```python
from build123d import *

# Parameters (mm, degrees)
SKETCH_1_W                    = 68
SKETCH_1_H                    = 75
EXTRUDE_1_DEPTH               = 14
SKETCH_2_R                    = 8.25
CUT_EXTRUDE_1_DEPTH           = 53.519044165
SKETCH_6_R                    = 35
CUT_EXTRUDE_3_DEPTH           = 8
HOLE_WIZARD_M2_2_D            = 2.4
HOLE_WIZARD_M2_2_DEPTH        = 6.35
HOLE_WIZARD_M2_2_CSINK_D      = 4.4
HOLE_WIZARD_M2_2_CSINK_ANGLE  = 90
HOLE_WIZARD_M2_2_TIP          = 0.721032743
HOLE_WIZARD_M2_5_1_AT_2_COUNT = 2
HOLE_WIZARD_M2_5_1_AT_2_PITCH = 18.5
HOLE_WIZARD_M2_5_2_D          = 2.05
HOLE_WIZARD_M2_5_2_DEPTH      = 6.35
HOLE_WIZARD_M2_5_2_TIP        = 0.615882135
SKETCH_19_R                   = 5
CUT_EXTRUDE_5_DEPTH           = 52.246951129
HOLE_WIZARD_M3_1_D            = 3.4
HOLE_WIZARD_M3_1_CSINK_D      = 6.3
HOLE_WIZARD_M3_1_CSINK_ANGLE  = 90


with BuildPart() as part:
    # 草圖1 → 填料-伸長1 (new body)
    with BuildSketch(Plane.XY):
        Rectangle(SKETCH_1_W, SKETCH_1_H)
    extrude(amount=EXTRUDE_1_DEPTH)

    # 草圖2 → 除料-伸長1 (cut, through all)
    with BuildSketch(Plane(origin=(0, 0, 0), x_dir=(-1, 0, 0), z_dir=(0, 0, -1))):
        with Locations((0, -5)):
            Circle(SKETCH_2_R)
    extrude(amount=-CUT_EXTRUDE_1_DEPTH, mode=Mode.SUBTRACT)

    # 草圖6 → 除料-伸長3 (cut)
    with BuildSketch(Plane(origin=(0, 0, 0), x_dir=(-1, 0, 0), z_dir=(0, 0, -1))):
        with Locations((0, -5)):
            Circle(SKETCH_6_R)
    extrude(amount=-CUT_EXTRUDE_3_DEPTH, mode=Mode.SUBTRACT)

    # M2 錐坑平頭螺釘的錐孔2
    with Locations(Plane(origin=(0, 0, 8), x_dir=(-1, 0, 0), z_dir=(0, 0, -1))):
        with Locations((-7.5, 2.5), (7.5, -12.5), (-7.5, -12.5), (7.5, 2.5)):
            CounterSinkHole(HOLE_WIZARD_M2_2_D / 2, HOLE_WIZARD_M2_2_CSINK_D / 2, depth=HOLE_WIZARD_M2_2_DEPTH, counter_sink_angle=HOLE_WIZARD_M2_2_CSINK_ANGLE)
            with Locations((0, 0, -(HOLE_WIZARD_M2_2_DEPTH + HOLE_WIZARD_M2_2_TIP / 2))):  # 118° drill point
                Cone(0, HOLE_WIZARD_M2_2_D / 2, HOLE_WIZARD_M2_2_TIP, mode=Mode.SUBTRACT)

    # 草圖13 → M2.5 螺紋孔1 (revolve, cut)
    with BuildSketch(Plane(origin=(-10.688129479, 24.3653944, 8), x_dir=(0, 1, 0), z_dir=(1, 0, 0))):
        Polygon((0, 0), (0, 6.965882135), (1.025, 6.35), (1.025, 0), align=None)
    hole_wizard_m2_5_1 = revolve(axis=Axis((-10.688129479, 24.3653944, 1.65), (0, 0, 1)), mode=Mode.SUBTRACT)

    # M2.5 螺紋孔1 at 2: M2.5 螺紋孔1 ×2
    with Locations(*[Vector(0.34202014332566283, -0.9396926207859105, 0) * (i * HOLE_WIZARD_M2_5_1_AT_2_PITCH) for i in range(1, HOLE_WIZARD_M2_5_1_AT_2_COUNT)]):
        add(hole_wizard_m2_5_1, mode=Mode.SUBTRACT)

    # 鏡射1: M2.5 螺紋孔1 across plane
    add(hole_wizard_m2_5_1.mirror(Plane(origin=(0, 0, 0), x_dir=(0, 0, 1), z_dir=(1, 0, 0))), mode=Mode.SUBTRACT)

    # 鏡射1 copy 1 sketch → 鏡射1 copy 1 (revolve, cut)
    with BuildSketch(Plane(origin=(4.360756827, 6.981080915, 8), x_dir=(0, 1, 0), z_dir=(-1, 0, 0))):
        Polygon((0, 0), (0, -6.965882135), (1.025, -6.35), (1.025, 0), align=None)
    revolve(axis=Axis((4.360756827, 6.981080915, 1.65), (0, 0, -1)), mode=Mode.SUBTRACT)

    # M2.5 螺紋孔2
    with Locations(Plane(origin=(0, 0, 8), x_dir=(-1, 0, 0), z_dir=(0, 0, -1))):
        with Locations((0, -17.75), (0, -36.25)):
            Hole(HOLE_WIZARD_M2_5_2_D / 2, depth=HOLE_WIZARD_M2_5_2_DEPTH)
            with Locations((0, 0, -(HOLE_WIZARD_M2_5_2_DEPTH + HOLE_WIZARD_M2_5_2_TIP / 2))):  # 118° drill point
                Cone(0, HOLE_WIZARD_M2_5_2_D / 2, HOLE_WIZARD_M2_5_2_TIP, mode=Mode.SUBTRACT)

    # 草圖19 → 除料-伸長5 (cut, through all)
    with BuildSketch(Plane(origin=(0, 0, 8), x_dir=(-1, 0, 0), z_dir=(0, 0, -1))):
        with Locations((-7.524443153, 15.673237657)):
            Circle(SKETCH_19_R)
        with Locations((7.524443153, 15.673237657)):
            Circle(SKETCH_19_R)
        with Locations((0, -27)):
            Circle(SKETCH_19_R)
    extrude(amount=-CUT_EXTRUDE_5_DEPTH, mode=Mode.SUBTRACT)

    # M3 錐坑平頭螺釘的錐孔1 (through all)
    with Locations(Plane.XY.offset(14)):
        with Locations((-29, 32.5), (-29, -32.5), (29, -32.5), (29, 32.5)):
            CounterSinkHole(HOLE_WIZARD_M3_1_D / 2, HOLE_WIZARD_M3_1_CSINK_D / 2, counter_sink_angle=HOLE_WIZARD_M3_1_CSINK_ANGLE)


solid = part.part
```
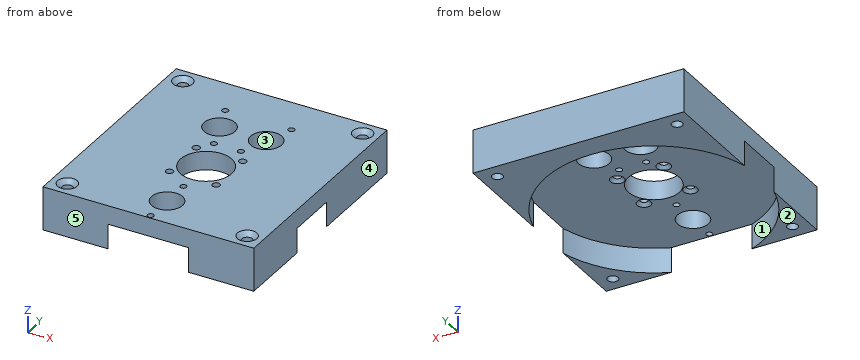
Input: part model. Units: mm. Frame: model coordinates. Face numbers are marked on the shaded views. A direction names the side the tool comes from. Give positions to 0.01 mm unless a question says otherwise; leave off trailing zeros. Order: outer loops, then holes, each group sorted by start corner. A loop starts at its lowest first (then second) coordinate and runs counter-clockwise, first axis right, second up. Notation, with made-up numbers: (76.25, 62) - (88.25, 62) arc R25 ccw to (88.25, 93) - close; hole circle Ø8 at (15, 81.25). An arc over 180 degrees is marked (long way). One line per item, written item: value.
1. Cut plane A-A, the plane z = 3.5. Output: boundary loops of the cut face in (x, y).
Determined:
outline: (-34, -37.5) - (-12.99, -37.5) arc R35 cw to (-34, -13.31) - close; (-34, 3.31) arc R35 cw to (34, 3.31) - (34, 37.5) - (-34, 37.5) - close; (12.99, -37.5) - (34, -37.5) - (34, -13.31) arc R35 cw to start; hole circle Ø3.4 at (-29, -32.5); hole circle Ø3.4 at (-29, 32.5); hole circle Ø3.4 at (29, -32.5); hole circle Ø3.4 at (29, 32.5)
2. Cut plane B-B, the plane y = -5. Output: boundary loops of the cut face in (x, z), and give its area (3 significant figures).
Determined:
outline: (-34, 8) - (-8.25, 8) - (-8.25, 14) - (-34, 14) - close; (8.25, 8) - (34, 8) - (34, 14) - (8.25, 14) - close
area: 309 mm2
3. Cut plane C-C, the plane y = 12.5. Output: boundary loops of the cut face in (x, z).
Determined:
outline: (-34, 0) - (-30.31, 0) - (-30.31, 8) - (-11.39, 8) - (-11.39, 14) - (-34, 14) - close; (-3.66, 8) - (3.66, 8) - (3.66, 14) - (-3.66, 14) - close; (11.39, 8) - (30.31, 8) - (30.31, 0) - (34, 0) - (34, 14) - (11.39, 14) - close
4. Pin query (flat end, axial travel): pin 1 Ø5.5 at (x, y) = (-29, 32.5) entering from +Z; pin 2 Ø4 at (x, y) = (-7.5, -12.5) entering from -Z; pin 3 Ø3 at (x, y) = (7.5, 2.5) entering from -Z; pin 4 Ø2.5 at (x, y) = (29, 32.5) entering from +Z. Return the tip coordinate at first contact, or that it passes through.
Determined:
pin 1: z = 13.6
pin 2: z = 8.2
pin 3: z = 8.7
pin 4: through
5. Cut plane D-D, the plane x = 24. Output: boundary loops of the cut face in (y, z), and give its area (3 significant figures).
Determined:
outline: (-37.5, 0) - (-30.48, 0) - (-30.48, 8) - (20.48, 8) - (20.48, 0) - (37.5, 0) - (37.5, 14) - (-37.5, 14) - close
area: 642 mm2
6. Line query: probe 1 along Y at (x, z) = (0, 9.7) (3 decimals); probe 2 along X at (y, z) = (7, 13.75); probe 3 along X at (y, z) = (-11.5, 8.5). Output: solid intervals per line, ascending.
Determined:
probe 1: -37.5 to -37.275, -35.225 to -32, -22 to -18.775, -16.725 to -13.25, 3.25 to 37.5
probe 2: -34 to -5.39, -3.34 to 3.34, 5.39 to 34
probe 3: -34 to -8.87, -6.13 to -5.08, 5.08 to 6.13, 8.87 to 34
7. Draft query along Y for the marked faces 3, 4 and 5. Return one class per face: released by +Y, released by -Y, zero draft, split by the parting line, or undercut.
Determined:
face 3: undercut
face 4: zero draft
face 5: released by -Y
8. Reachability of the marked faces 1 and 2 from +Z, -Z, +X, -X, +Y, -Y: full face, straight path, thin tool, end or side. Return the list, or none.
Determined:
face 1: -Z
face 2: -Z, +X, -X, +Y, -Y
